```python
from build123d import *

# Parameters (mm, degrees)
BOSS_EXTRUDE1_DEPTH = 1


with BuildPart() as part:
    # Sketch2 → Boss-Extrude1 (new body)
    with BuildSketch(Plane.XY):
        with BuildLine():
            Line((-4.401739713, -3.903473849), (-4.401739713, -3.405207986))
            Line((-4.401739713, -3.405207986), (-4.401739713, -2.906942122))
            ThreePointArc((-4.401739713, -2.906942122), (-4.884506928, -1.991787406), (-5.179346001, -1))
            ThreePointArc((-5.179346001, -1), (-5.738651784, -0.642015565), (-5.908333333, 0))
            ThreePointArc((-5.908333333, 0), (0, 5.275), (5.908333333, 0))
            ThreePointArc((5.908333333, 0), (5.738651784, -0.642015565), (5.179346001, -1))
            ThreePointArc((5.179346001, -1), (4.884506928, -1.991787406), (4.401739713, -2.906942122))
            Line((4.401739713, -2.906942122), (4.401739713, -3.405207986))
            Line((4.401739713, -3.405207986), (4.401739713, -3.903473849))
            ThreePointArc((4.401739713, -3.903473849), (4.543651106, -4.41534116), (4.849574008, -4.849574008))
            Line((4.849574008, -4.849574008), (5.073491155, -5.073491155))
            ThreePointArc((5.073491155, -5.073491155), (0, 7.175), (-5.073491155, -5.073491155))
            Line((-5.073491155, -5.073491155), (-4.849574008, -4.849574008))
            ThreePointArc((-4.849574008, -4.849574008), (-4.543651106, -4.41534116), (-4.401739713, -3.903473849))
        make_face()
    extrude(amount=BOSS_EXTRUDE1_DEPTH)


solid = part.part
```
Read the model definition and answer for the solid it produces. Units are mm, in the model's axes. A direction names the side the tool comes from. Coordinates: 2 decimals unless noted, no trailing zeros. Loops run counter-clockwise (first coordinate to the right, second up) from the corner with the lowest first, then second, coordinate; pieces in that order, holes last.
(1) The part is cut by section B-B (y = -0.5). Determine the outline of the cut face in (x, z), and give its area (3 significant figures).
Solution:
outline: (-7.16, 0) - (-5.82, 0) - (-5.82, 1) - (-7.16, 1) - close; (5.82, 0) - (7.16, 0) - (7.16, 1) - (5.82, 1) - close
area: 2.67 mm2
(2) The mould has two halves that part along Y. Classify faces 4 (the face through (-5.733, -0.65, 0.493)), 5 (the face through (4.402, -3.4, 0.5)), 6 (the face through (0.24, 7.17, 0.49)): released by +Y, released by -Y, zero draft, split by the parting line, or undercut.
Solution:
face 4: undercut
face 5: zero draft
face 6: split by the parting line
(3) A tool of negligible diameter and unlimited length cuts with its end or side. For faces 1 (the face through (4.89, -1.98, 0.49)), 2 (the face through (4.54, -4.41, 0.49)), 3 (the face through (0, 6, 0)), from which of +Z, -Z, +X, -X, +Y, -Y can it reach the whole face along a straight path? Write none if from no direction.
Solution:
face 1: +Z, -Z
face 2: +Z, -Z, -Y
face 3: -Z, +X, -X, +Y, -Y
(4) The part is cut by section C-C (x = 0). Determine the outline of the cut face in (y, z) (3 decimals).
Solution:
outline: (5.275, 0) - (7.175, 0) - (7.175, 1) - (5.275, 1) - close
(5) Consider line 1 along X through (y, z) = (1, 0.45); line 2 along Y through (x, z) = (5.5, 0.55); line 3 along X through (y, z) = (-2.5, 0.7). Determine where each line is inside the solid, lowest interval first.
Solution:
line 1: x = -7.1 to -5.71, 5.71 to 7.1
line 2: y = -4.61 to -0.87, 1.59 to 4.61
line 3: x = -6.73 to -4.64, 4.64 to 6.73
(6) The part is cut by section D-D (y = 2.75). Determine the outline of the cut face in (x, z).
Solution:
outline: (-6.63, 0) - (-4.86, 0) - (-4.86, 1) - (-6.63, 1) - close; (4.86, 0) - (6.63, 0) - (6.63, 1) - (4.86, 1) - close
